Model file for the job. Use its own axes, mm. A direction names the side the tool comes from. Give positions to 0.01 mm unless a question says otherwise; leave off trailing zeros. Write each loop counter-clockwise with the first axis right and the second up, starting at its lowest first coordinate (ties: lowest second). Pieces come first, ordered by that corner, then holes. Notation, with made-up numbers: (86.25, 12) - (102.25, 12) arc R26 ccw to (102.25, 44) - close; hole circle Ø8 at (65, -26). An arc over 180 degrees is marked (long way). One line per item, written item: value. Start each with the question number.
(1) Drop flat-ended pins along their axis: P1, Ø9, axis at x = 16.5, y = 25, coming from the +Z side; P2, Ø24, axis at x = 59, y = 27, coming from the +Z side; P3, Ø3, axis at x = -72.25, y = -44, coming from the +Z side. Give the stop position or say it passes through.
(2) Cut at A-A, the plane x = -58.25. List the corners of the cut face in (y, z).
(3) Probe L1, parallel to Y at x = 19.45, z = 0.4; L2, parallel to Y at x = 58.3, z = 0.55; L3, parallel to X at y = 3.5, z = 0.4. List the from-to ranges inside material, lowest first.
(4) Cut at B-B, the plane z = 0.5. State how many separate pieces and enclosed holes the cut face has, and give its area (3 significant figures).
(5) Cut at C-C, the plane y = 9. List the corners of the cut face in (x, z), and give its area (3 significant figures).
(6) Mould opens along Y. For faces 1 (the face through (-1, 1, -0.6)), 2 (the face through (72.607, 34.506, 0.444)) say: pulls with the +Y half, pulls with the -Y half, needs draft (parallel to the pull), parting line crosses it, or undercut.
(7) 3-axis set-ups, long thin cutter, end or side, ignore diameter. For faces 3 (the face through (-74.234, -45.521, 0.16)), 4 (the face through (-5.093, -25.494, 0.444)): which of +Z, -Z, +X, -X, +Y, -Y reach the whole face in a straight line?
(8) Cut at D-D, the plane x = 19.45. List the corners of the cut face in (y, z).
from build123d import *

# Parameters (mm, degrees)
F0_W     = 152.5
F0_H     = 96
F0_R     = 15
F1_DEPTH = 0.9
F2_DEPTH = 0.6
F3_R     = 2.5
F4_DEPTH = 1.501


# Not quite as in the source:
# - a feature names something its author has since deleted; it is built from what else it names


with BuildPart() as f1:
    # F0 (on Top) → F1 (new body)
    with BuildSketch(Plane.XY):
        Rectangle(F0_W, F0_H)
        with Locations((-58.25, -30)):
            Circle(F0_R, mode=Mode.SUBTRACT)
        with Locations((-19.4, -30)):
            Circle(F0_R, mode=Mode.SUBTRACT)
        with Locations((19.45, -30)):
            Circle(F0_R, mode=Mode.SUBTRACT)
        with Locations((58.3, -30)):
            Circle(F0_R, mode=Mode.SUBTRACT)
        with Locations((-38.85, 0)):
            Circle(F0_R, mode=Mode.SUBTRACT)
        with Locations((-58.25, 30)):
            Circle(F0_R, mode=Mode.SUBTRACT)
        with Locations((-19.4, 30)):
            Circle(F0_R, mode=Mode.SUBTRACT)
        Circle(F0_R, mode=Mode.SUBTRACT)
        with Locations((38.85, 0)):
            Circle(F0_R, mode=Mode.SUBTRACT)
        with Locations((19.45, 30)):
            Circle(F0_R, mode=Mode.SUBTRACT)
        with Locations((58.3, 30)):
            Circle(F0_R, mode=Mode.SUBTRACT)
    extrude(amount=F1_DEPTH)

    # F0 (on Top) → F2 (join)
    with BuildSketch(Plane.XY):
        Rectangle(F0_W, F0_H)
        with Locations((-58.25, -30)):
            Circle(F0_R, mode=Mode.SUBTRACT)
        with Locations((-19.4, -30)):
            Circle(F0_R, mode=Mode.SUBTRACT)
        with Locations((19.45, -30)):
            Circle(F0_R, mode=Mode.SUBTRACT)
        with Locations((58.3, -30)):
            Circle(F0_R, mode=Mode.SUBTRACT)
        with Locations((-38.85, 0)):
            Circle(F0_R, mode=Mode.SUBTRACT)
        with Locations((-58.25, 30)):
            Circle(F0_R, mode=Mode.SUBTRACT)
        with Locations((-19.4, 30)):
            Circle(F0_R, mode=Mode.SUBTRACT)
        Circle(F0_R, mode=Mode.SUBTRACT)
        with Locations((38.85, 0)):
            Circle(F0_R, mode=Mode.SUBTRACT)
        with Locations((19.45, 30)):
            Circle(F0_R, mode=Mode.SUBTRACT)
        with Locations((58.3, 30)):
            Circle(F0_R, mode=Mode.SUBTRACT)
        with Locations((-58.25, -30)):
            Circle(F0_R)
        with Locations((-38.85, 0)):
            Circle(F0_R)
        with Locations((-58.25, 30)):
            Circle(F0_R)
        with Locations((-19.4, 30)):
            Circle(F0_R)
        with Locations((19.45, 30)):
            Circle(F0_R)
        Circle(F0_R)
        with Locations((38.85, 0)):
            Circle(F0_R)
        with Locations((19.45, -30)):
            Circle(F0_R)
        with Locations((58.3, -30)):
            Circle(F0_R)
        with Locations((58.3, 30)):
            Circle(F0_R)
        with Locations((-19.4, -30)):
            Circle(F0_R)
    extrude(amount=-F2_DEPTH)

    # F3 (on face) → F4 (cut, through all)
    with BuildSketch(Plane.XY.offset(0.9)):
        with Locations((-72.25, 44)):
            Circle(F3_R)
        with Locations((72.25, 44)):
            Circle(F3_R)
        with Locations((-72.25, -44)):
            Circle(F3_R)
        with Locations((72.25, -44)):
            Circle(F3_R)
        with Locations((-19.425, 0)):
            Circle(F3_R)
        with Locations((19.425, 0)):
            Circle(F3_R)
    extrude(amount=-F4_DEPTH, mode=Mode.SUBTRACT)


solid = f1.part
Answers follow:
1. P1: stops at z = 0
1. P2: stops at z = 0.9
1. P3: passes through
2. outline: (-48, -0.6) - (48, -0.6) - (48, 0.9) - (45, 0.9) - (45, 0) - (15, 0) - (15, 0.9) - (-15, 0.9) - (-15, 0) - (-45, 0) - (-45, 0.9) - (-48, 0.9) - close
3. L1: y = -48 to -45, -15 to -2.5, 2.5 to 15, 45 to 48
3. L2: y = -48 to -45, -15 to 15, 45 to 48
3. L3: x = -76.25 to -53.44, -24.26 to -14.59, 14.59 to 24.26, 53.44 to 76.25
4. separate pieces: 1
4. enclosed holes: 17
4. area: 6,750 mm²
5. outline: (-76.25, -0.6) - (76.25, -0.6) - (76.25, 0.9) - (50.85, 0.9) - (50.85, 0) - (26.85, 0) - (26.85, 0.9) - (12, 0.9) - (12, 0) - (-12, 0) - (-12, 0.9) - (-26.85, 0.9) - (-26.85, 0) - (-50.85, 0) - (-50.85, 0.9) - (-76.25, 0.9) - close
5. area: 164 mm²
6. face 1: needs draft
6. face 2: undercut
7. face 3: +Z, -Z
7. face 4: +Z
8. outline: (-48, -0.6) - (-2.5, -0.6) - (-2.5, 0.9) - (-15, 0.9) - (-15, 0) - (-45, 0) - (-45, 0.9) - (-48, 0.9) - close; (2.5, -0.6) - (48, -0.6) - (48, 0.9) - (45, 0.9) - (45, 0) - (15, 0) - (15, 0.9) - (2.5, 0.9) - close
